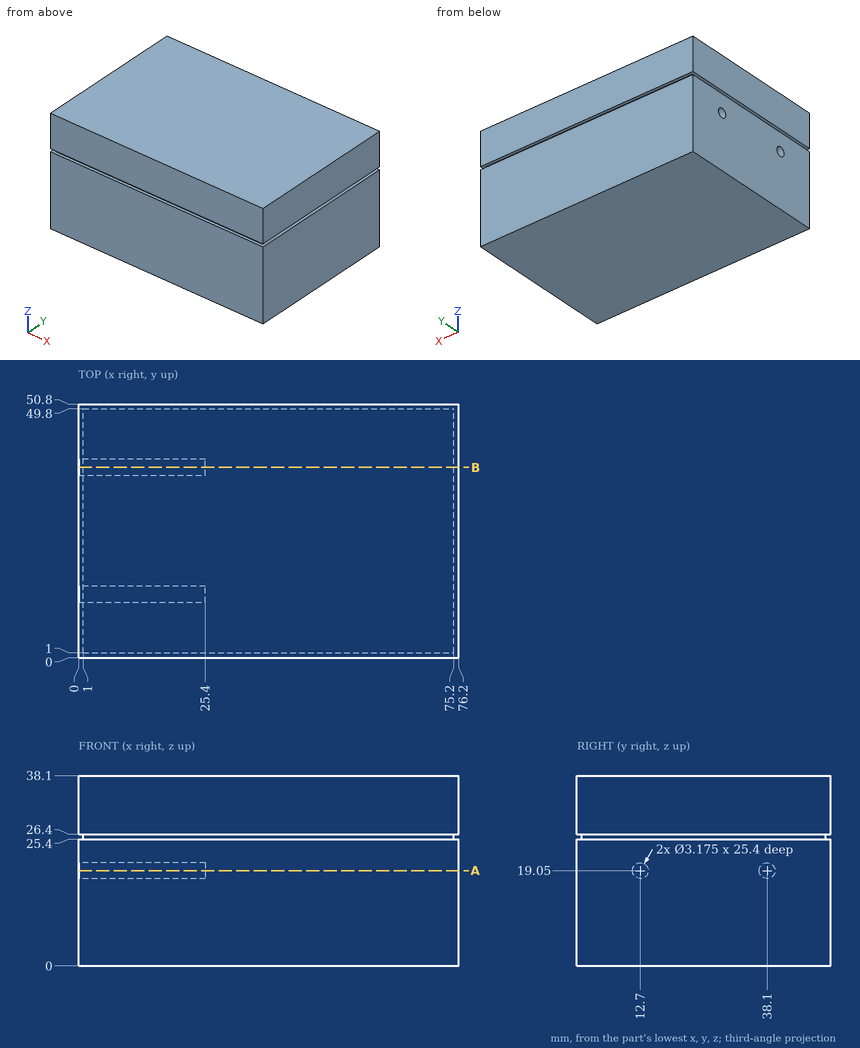
Can you work these out from the drawing? Everything is in mm from the part's minimum corner. Round coordinates to 2 decimals unless told otherwise and drop trailing zeros. Loops run counter-clockwise (first coordinate to the right, second up) from the corner with the lowest first, then second, coordinate; pieces in that order, holes last. Notation, with made-up numbers: (-1.5, 67.25) - (22.5, 67.25) arc R24 cw to (22.5, 80.25) - close; hole circle Ø3 at (83.25, 0). An arc over 180 degrees is marked (long way). One line per question, with ' | ' between items. Start each with the question number.
Q1. Will this pin go through, and if not, where does the flat tip stop? pin 1 (1 mm diameter, centred on y = 13, z = 19.5, fed in from -X).
Q2. I want a section at B-B (y = 38.1). Write out the boundary of the cut face in (x, z).
Q3. Please list where these lines run through material, in increasing order: line 1 (Y direction, x = 16, z = 19); line 2 (Z direction, x = 20, y = 12.7). Write a range as [from, to].
Q4. I want a section at A-A (z = 19.05). Write out the boundary of the cut face in (x, y).
Response values:
1) pin 1: stops at x = 25.4
2) outline: (0, 0) - (76.2, 0) - (76.2, 25.4) - (75.2, 25.4) - (75.2, 26.4) - (76.2, 26.4) - (76.2, 38.1) - (0, 38.1) - (0, 26.4) - (1, 26.4) - (1, 25.4) - (0, 25.4) - (0, 20.64) - (25.4, 20.64) - (25.4, 17.46) - (0, 17.46) - close
3) line 1: y = [0, 11.11], [14.29, 36.51], [39.69, 50.8] | line 2: z = [0, 17.46], [20.64, 38.1]
4) outline: (0, 0) - (76.2, 0) - (76.2, 50.8) - (0, 50.8) - (0, 39.69) - (25.4, 39.69) - (25.4, 36.51) - (0, 36.51) - (0, 14.29) - (25.4, 14.29) - (25.4, 11.11) - (0, 11.11) - close
